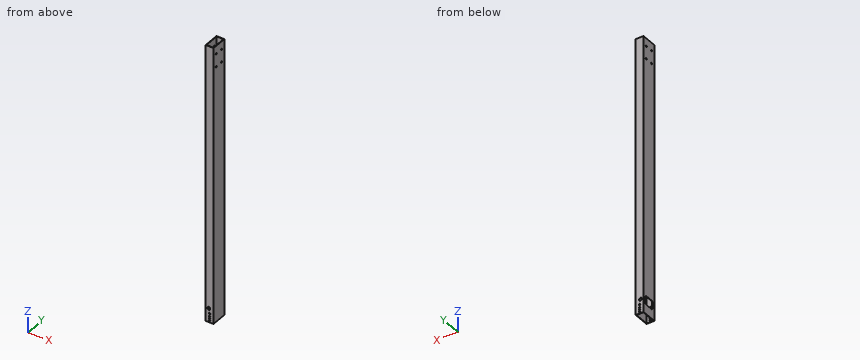
Autodesk Inventor part; units mm, degrees
ref_plane "YZ Plane" through (0, 0, 0) normal (1, 0, 0) x (0, 1, 0)
ref_plane "XZ Plane" through (0, 0, 0) normal (0, 1, 0) x (-1, 0, 0)
ref_plane "XY Plane" through (0, 0, 0) normal (0, 0, 1) x (1, 0, 0)
sketch "Sketch1" plane through (0, 0, 0) normal (0, 0, 1) x (1, 0, 0)
  line L0 (-12.7, -25.4) -> (12.7, -25.4)
  line L1 (12.7, -25.4) -> (12.7, 25.4)
  line L2 (12.7, 25.4) -> (-12.7, 25.4)
  line L3 (-12.7, 25.4) -> (-12.7, -25.4)
  line L4 (-12.7, -25.4) -> (12.7, 25.4) construction
  line L5 (12.7, -25.4) -> (-12.7, 25.4) construction
  line L6 (-11.1125, 23.8125) -> (11.1125, 23.8125)
  line L7 (11.1125, 23.8125) -> (11.1125, -23.8125)
  line L8 (11.1125, -23.8125) -> (-11.1125, -23.8125)
  line L9 (-11.1125, -23.8125) -> (-11.1125, 23.8125)
  point P0 (0, 0)
  dimension "width" = 25.4
  dimension "height" = 50.8
  dimension "thickness" = 1.5875
extrude "Extrusion1" add sketch "Sketch1" along normal mid plane 889
sketch "Sketch2" plane through (-12.7, 25.4, 444.5) normal (0, 1, 0) x (1, 0, 0)
  line L0 (0, 889) -> (0, 0)
  line L1 (0, 889) -> (25.4, 889)
  point P0 (12.7, 444.5)
  point P1 (12.7, 882.65)
  point P2 (12.7, 876.3)
  point P3 (12.7, 869.95)
  point P4 (12.7, 889)
  point P5 (12.7, 860.425)
  dimension "d5" = 12.7
  dimension "d6" = 6.35
  dimension "d7" = 6.35
  dimension "d8" = 6.35
  dimension "d45" = 9.525
hole "Hole1" at (0, 25.4, -438.15) at (0, 25.4, -431.8) at (0, 25.4, -425.45) at (0, 25.4, -415.925) direction (0, -1, 0) diameter 5.1054 end through all
sketch "Sketch4" plane through (-12.7, 25.4, 444.5) normal (0, 1, 0) x (1, 0, 0)
  circle A0 centre (9.9314, 844.55) radius 10.3124 construction
  line L0 (0, 889) -> (0, 0) construction
  circle A1 centre (12.7, 869.95) radius 2.5527 construction
  point P0 (12.7, 444.5)
  dimension "d27" = 20.6248
  dimension "d28" = 9.9314
  dimension "d29" = 25.4
hole "Hole3" at (-2.7686, 25.4, -400.05) direction (0, -1, 0) diameter 9.525 end through all
sketch "Sketch5" plane through (-12.7, -25.4, 444.5) normal (-1, 0, 0) x (0, 0, 1)
  line L0 (-830.58, 41.275) -> (-858.52, 41.275)
  line L1 (-858.52, 41.275) -> (-858.52, 9.525)
  line L2 (-858.52, 9.525) -> (-830.58, 9.525)
  line L3 (-830.58, 9.525) -> (-830.58, 41.275)
  line L4 (-830.58, 41.275) -> (-858.52, 9.525) construction
  line L5 (-858.52, 41.275) -> (-830.58, 9.525) construction
  line L6 (0, 0) -> (-889, 0)
  line L7 (-889, 0) -> (-889, 50.8)
  point P0 (-444.5, 25.4)
  point P1 (-844.55, 25.4)
  point P2 (-858.52, 25.4)
  point P3 (-889, 25.4)
  point P4 (-889, 25.4)
  dimension "d37" = 27.94
  dimension "d38" = 31.75
  dimension "d43" = 44.45
extrude "Extrusion2" cut sketch "Sketch5" against normal blind 1.5875
fillet "Fillet1" radius 3.302 4 edges at (-11.9062, -15.875, -414.02) (-11.9062, 15.875, -414.02) (-11.9062, 15.875, -386.08) (-11.9062, -15.875, -386.08)
sketch "Sketch6" plane through (12.7, -25.4, 444.5) normal (1, 0, 0) x (0, 0, -1)
  line L0 (889, 50.8) -> (0, 50.8) construction
  line L1 (0, 0) -> (0, 50.8) construction
  line L2 (889, 0) -> (0, 0) construction
  line L3 (889, 50.8) -> (889, 0) construction
  point P0 (444.5, 25.4)
  point P1 (25.4, 38.1)
  point P2 (25.4, 12.7)
  point P3 (66.675, 38.1)
  point P4 (66.675, 12.7)
  dimension "d46" = 25.4
  dimension "d47" = 12.7
  dimension "d48" = 12.7
  dimension "d49" = 41.275
hole "Hole4" at (12.7, 12.7, 419.1) at (12.7, -12.7, 419.1) at (12.7, 12.7, 377.825) at (12.7, -12.7, 377.825) direction (-1, 0, 0) diameter 5.1054 end through all
properties part number "EL2-001" material "Aluminum 6061"
Here's how the part is built. I have some questions about the finished solid (model axes, mm). Round coordinates to 2 decimals unless told otherwise and drop trailing zeros. Order: outer loops, then holes, each group sorted by start corner. A loop starts at its lowest first (then second) coordinate and runs counter-clockwise, first axis right, second up. Notation, with made-up numbers: (11, 35) -> (54, 35) arc R5 cw to (54, 44) -> close; hole circle Ø10 at (73, 18). An arc over 180 degrees is marked (long way). Use a Markdown table: item, result. Add a question column.
(1) I need wall thicknesses on line 1 along Z through (x, y) = (11.7, -12.7); line 2 along Z through (x, y) = (-11.7, -12.7); line 3 along X through (y, z) = (9, 72). Which ranges of each line are inside material? Lowest first, please.
(2) Suppose I cut it at A-A, the plane z = 295.5. Please give me the cut outline in (x, y).
(3) For pin 1 Ø12 at (x, y) = (-7, -14.5) entering from -Z; pin 2 Ø4 at (y, z) = (12.7, 377.825) entering from +X, each with a flat end and sliding along its axis, tell me the tip position at first contact or that it passes through.
Verdict:
| question | item | result |
|---|---|---|
| 1 | line 1 | -444.5 to 375.27, 380.38 to 416.55, 421.65 to 444.5 |
| 1 | line 2 | -444.5 to -414.02, -386.08 to 375.27, 380.38 to 416.55, 421.65 to 444.5 |
| 1 | line 3 | -12.7 to -11.11, 11.11 to 12.7 |
| 2 | outline | (-12.7, -25.4) -> (12.7, -25.4) -> (12.7, 25.4) -> (-12.7, 25.4) -> close; hole (-11.11, -23.81) -> (11.11, -23.81) -> (11.11, 23.81) -> (-11.11, 23.81) -> close |
| 3 | pin 1 | z = -444.5 |
| 3 | pin 2 | through |
